from build123d import *

# Parameters (mm, degrees)
SKETCH1_W           = 41.4782
SKETCH1_H           = 17.78
SKETCH1_R           = 4.445
SKETCH1_R_2         = 1.5875
BOSS_EXTRUDE1_DEPTH = 6.35
SKETCH2_W           = 6.35
SKETCH2_H           = 6.35
BOSS_EXTRUDE2_DEPTH = 0.254
SKETCH3_W           = 6.35
SKETCH3_H           = 25.4
BOSS_EXTRUDE3_DEPTH = 12.7
SKETCH4_W           = 12.7
SKETCH4_H           = 6.35
BOSS_EXTRUDE4_DEPTH = 127
SKETCH5_R           = 1.5875
CUT_EXTRUDE1_DEPTH  = 7.35
SKETCH6_W           = 21.59
SKETCH6_H           = 17.78
CUT_EXTRUDE2_DEPTH  = 26.4
FILLET1_R           = 3.175


with BuildPart() as part:
    # Sketch1 → Boss-Extrude1 (new body)
    with BuildSketch(Plane(origin=(0, 0, 0), x_dir=(1, 0, 0), z_dir=(0, 1, 0))):
        Rectangle(SKETCH1_W, SKETCH1_H)
        with Locations((-8.0391, 0)):
            Circle(SKETCH1_R, mode=Mode.SUBTRACT)
        with Locations((13.6271, 0)):
            Circle(SKETCH1_R_2, mode=Mode.SUBTRACT)
        with Locations((8.0391, 0)):
            Circle(SKETCH1_R_2, mode=Mode.SUBTRACT)
    extrude(amount=BOSS_EXTRUDE1_DEPTH)

    # Sketch2 → Boss-Extrude2 (add)
    with BuildSketch(Plane(origin=(0, 0, -8.89), x_dir=(-1, 0, 0), z_dir=(0, 0, -1))):
        with Locations((-17.5641, 3.175)):
            Rectangle(SKETCH2_W, SKETCH2_H)
    extrude(amount=BOSS_EXTRUDE2_DEPTH)

    # Sketch3 → Boss-Extrude3 (add)
    with BuildSketch(Plane(origin=(0, 0, -9.144), x_dir=(-1, 0, 0), z_dir=(0, 0, -1))):
        with Locations((-17.5641, -6.35)):
            Rectangle(SKETCH3_W, SKETCH3_H)
    extrude(amount=BOSS_EXTRUDE3_DEPTH)

    # Sketch4 → Boss-Extrude4 (add)
    with BuildSketch(Plane(origin=(20.7391, 0, 0), x_dir=(0, 0, -1), z_dir=(1, 0, 0))):
        with Locations((15.494, -15.875)):
            Rectangle(SKETCH4_W, SKETCH4_H)
    extrude(amount=BOSS_EXTRUDE4_DEPTH)

    # Sketch5 → Cut-Extrude1 (cut, through all)
    with BuildSketch(Plane(origin=(0, -12.7, 0), x_dir=(1, 0, 0), z_dir=(0, 1, 0))):
        with Locations((33.4391, 18.669)):
            Circle(SKETCH5_R)
        with Locations((33.4391, 12.319)):
            Circle(SKETCH5_R)
        with Locations((46.1391, 12.319)):
            Circle(SKETCH5_R)
        with Locations((46.1391, 18.669)):
            Circle(SKETCH5_R)
        with Locations((58.8391, 12.319)):
            Circle(SKETCH5_R)
        with Locations((58.8391, 18.669)):
            Circle(SKETCH5_R)
        with Locations((71.5391, 12.319)):
            Circle(SKETCH5_R)
        with Locations((71.5391, 18.669)):
            Circle(SKETCH5_R)
        with Locations((84.2391, 12.319)):
            Circle(SKETCH5_R)
        with Locations((84.2391, 18.669)):
            Circle(SKETCH5_R)
        with Locations((96.9391, 12.319)):
            Circle(SKETCH5_R)
        with Locations((96.9391, 18.669)):
            Circle(SKETCH5_R)
        with Locations((109.6391, 12.319)):
            Circle(SKETCH5_R)
        with Locations((109.6391, 18.669)):
            Circle(SKETCH5_R)
        with Locations((122.3391, 12.319)):
            Circle(SKETCH5_R)
        with Locations((122.3391, 18.669)):
            Circle(SKETCH5_R)
        with Locations((135.0391, 12.319)):
            Circle(SKETCH5_R)
        with Locations((135.0391, 18.669)):
            Circle(SKETCH5_R)
    extrude(amount=-CUT_EXTRUDE1_DEPTH, mode=Mode.SUBTRACT)

    # Sketch6 → Cut-Extrude2 (cut, through all)
    with BuildSketch(Plane(origin=(0, 6.35, 0), x_dir=(1, 0, 0), z_dir=(0, 1, 0))):
        with Locations((-9.9441, 0)):
            Rectangle(SKETCH6_W, SKETCH6_H)
    extrude(amount=-CUT_EXTRUDE2_DEPTH, mode=Mode.SUBTRACT)

    # Fillet1
    fillet1_edges = [part.edges().sort_by_distance(p)[0] for p in [
        (0.8509, 3.175, 8.89),
        (0.8509, 3.175, -8.89),
        (14.3891, -19.05, -15.494),
        (17.5641, 6.35, -21.844),
        (20.7391, -12.7, -15.494),
        (147.7391, -15.875, -9.144),
        (147.7391, -15.875, -21.844),
        (20.7391, 3.175, 8.89),
    ]]
    fillet(fillet1_edges, radius=FILLET1_R)


solid = part.part
Model file for the job. Use its own axes, mm. A direction names the side the tool comes from. Give positions to 0.01 mm unless a question says otherwise; leave off trailing zeros. Write each loop counter-clockwise with the first axis right and the second up, starting at its lowest first coordinate (ties: lowest second). Pieces come first, ordered by that corner, then holes. Notation, with made-up numbers: M -30.75,37 L -1.75,37 A20 ccw -1.75,67 Z; hole C -2.5,24.25 d2. An arc over 180 degrees is marked long. One line per item, written item: value. Start each with the question number.
Q1. Saw through at A-A, the plane z = 0. Write the cut outline in (x, y).
Q2. Saw through at B-B, the plane y = -6. Write the cut outline in (x, z), plus the area to 3 significant figures.
Q3. Drop flat-ended pins along their axis: pin 1 Ø1 at (y, z) = (-8, -17.5) entering from -X; pin 2 Ø4 at (x, z) = (96.94, -18.67) entering from +Y; pin 3 Ø1.5 at (y, z) = (0.5, -5.5) entering from +X. Give the stop position or say it passes through.
Q4. Two-plate mould, pull along Z, no slides. Class faces 4 (the cylindrical face through (1.76, 3.13, -7.94)), 5 (the cylindrical face through (44.97, -15.83, -19.74)), 6 (the flat face through (64, -14, -9.144)), 7 (the cylindrical face through (96.732, -15.831, -20.243)): +Z half, -Z half, draft (parallel to the pull), parting line (faces both ways), or undercut.
Q5. 3-axis set-ups, long thin cutter, end or side, ignore diameter. For faces 1 (the cylindrical face through (21.7, -11.8, -15.6)), 2 (the flat face through (9, 3, -8.89)), 3 (the flat face through (11, 0, 0)): which of +Z, -Z, +X, -X, +Y, -Y reach the whole face in a straight line?
Q6. Probe probe 1 along Z at (x, y) = (128, -15.25); probe 2 along X at (y, z) = (-3.25, -18); probe 3 along Y at (x, z) = (120, -19.5). List the from-to ranges inside material, lowest first. Write a range as [from, to].
Q7. Saw through at C-C, the plane x = 130.5. Write the cut outline in (y, z).
Output values:
1. outline: M 0.85,0 L 6.45,0 L 6.45,6.35 L 0.85,6.35 Z; M 9.63,0 L 12.04,0 L 12.04,6.35 L 9.63,6.35 Z; M 15.21,0 L 20.74,0 L 20.74,6.35 L 15.21,6.35 Z
2. outline: M 14.39,-21.84 L 20.74,-21.84 L 20.74,-9.14 L 14.39,-9.14 Z
2. area: 80.6 mm²
3. pin 1: stops at x = 14.39
3. pin 2: stops at y = -12.7
3. pin 3: stops at x = 20.74
4. face 4: -Z half
4. face 5: undercut
4. face 6: +Z half
4. face 7: undercut
5. face 1: +Z, -Z, +X, +Y
5. face 2: -Z, -X, +Y, -Y
5. face 3: +Z, +X, -X, -Y
6. probe 1: z = [-21.84, -9.14]
6. probe 2: x = [14.39, 20.74]
6. probe 3: y = [-19.05, -12.7]
7. outline: M -19.05,-21.84 L -12.7,-21.84 L -12.7,-9.14 L -19.05,-9.14 Z
